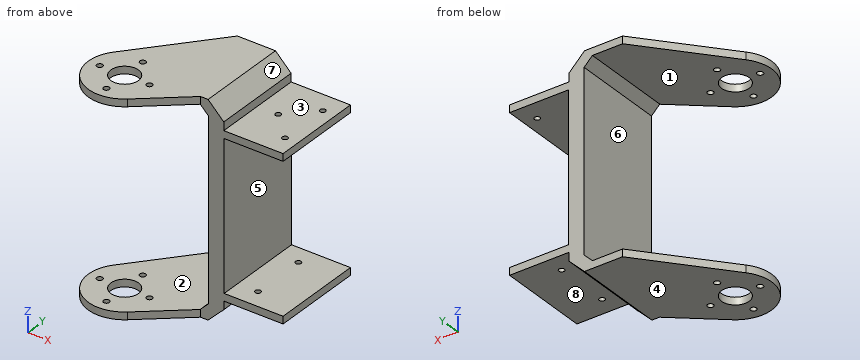
from build123d import *

# Parameters (mm, degrees)
EXTRUDE_1_DEPTH                 = 25
CUT_EXTRUDE_1_REACH             = 54.692
SKETCH_2_R                      = 0.75
CUT_EXTRUDE_1_DIRECTION_2_DEPTH = 53.691808082
EXTRUDE_2_DEPTH                 = 25
EXTRUDE_3_DEPTH                 = 2
CUT_EXTRUDE_4_DEPTH             = 73.027407742
CUT_EXTRUDE_4_DEPTH_BACK        = 73.027407742
SKETCH_6_R                      = 3.75
SKETCH_6_R_2                    = 0.8
CUT_EXTRUDE_START               = -44
SKETCH_8_R                      = 0.75
CUT_EXTRUDE_5_DEPTH             = 2


with BuildPart() as part:
    # 草图1 → 凸台-拉伸1 (new body)
    with BuildSketch(Plane(origin=(0, 0, 0), x_dir=(1, 0, 0), z_dir=(0, 1, 0))):
        Polygon((14.677419355, 32.709677419), (-1.322580645, 32.709677419), (-1.322580645, -7.290322581), (14.677419355, -7.290322581), (14.677419355, -9.290322581), (-3.322580645, -9.290322581), (-3.322580645, 34.709677419), (14.677419355, 34.709677419), align=None)
    extrude(amount=EXTRUDE_1_DEPTH)

    # 草图2 → 切除-拉伸1 (cut, up to next)
    with BuildSketch(Plane.XY.offset(9.290322581), mode=Mode.PRIVATE) as cut_extrude_1_sk1:
        with Locations(Location((4.195809336, 12.5, 0), (0, 0, 180))):
            Circle(SKETCH_2_R)
    cut_extrude_1_tool1 = extrude(cut_extrude_1_sk1.sketch, amount=-CUT_EXTRUDE_1_REACH, mode=Mode.PRIVATE) & part.part
    # 草图2 → 切除-拉伸1 (cut, up to next)
    with BuildSketch(Plane.XY.offset(9.290322581), mode=Mode.PRIVATE) as cut_extrude_1_sk2:
        with Locations(Location((11.195809336, 19.5, 0), (0, 0, 180))):
            Circle(SKETCH_2_R)
    cut_extrude_1_tool2 = extrude(cut_extrude_1_sk2.sketch, amount=-CUT_EXTRUDE_1_REACH, mode=Mode.PRIVATE) & part.part
    # 草图2 → 切除-拉伸1 (cut, up to next)
    with BuildSketch(Plane.XY.offset(9.290322581), mode=Mode.PRIVATE) as cut_extrude_1_sk3:
        with Locations(Location((11.195809336, 5.5, 0), (0, 0, 180))):
            Circle(SKETCH_2_R)
    cut_extrude_1_tool3 = extrude(cut_extrude_1_sk3.sketch, amount=-CUT_EXTRUDE_1_REACH, mode=Mode.PRIVATE) & part.part
    add(cut_extrude_1_tool1.solids().sort_by_distance((4.195809, 12.5, 9.290323))[0], mode=Mode.SUBTRACT)
    add(cut_extrude_1_tool2.solids().sort_by_distance((11.195809, 19.5, 9.290323))[0], mode=Mode.SUBTRACT)
    add(cut_extrude_1_tool3.solids().sort_by_distance((11.195809, 5.5, 9.290323))[0], mode=Mode.SUBTRACT)

    # 草图2 → 切除-拉伸1 direction 2 (cut)
    with BuildSketch(Plane.XY.offset(9.290322581)):
        with Locations(Location((4.195809336, 12.5, 0), (0, 0, 180))):
            Circle(SKETCH_2_R)
        with Locations(Location((11.195809336, 19.5, 0), (0, 0, 180))):
            Circle(SKETCH_2_R)
        with Locations(Location((11.195809336, 5.5, 0), (0, 0, 180))):
            Circle(SKETCH_2_R)
    extrude(amount=CUT_EXTRUDE_1_DIRECTION_2_DEPTH, mode=Mode.SUBTRACT)

    # 草图5 → 凸台-拉伸2 (add)
    with BuildSketch(Plane(origin=(0, 25, 0), x_dir=(1, 0, 0), z_dir=(0, 1, 0))):
        Polygon((-3.682839685, 39.209677419), (-1.432839685, 36.959677419), (-1.432839685, 34.709677419), (-3.322580645, 34.709677419), (-3.322580645, 32.459677419), (-3.322580645, 12.709677419), (-5.572580645, 12.709677419), (-5.572580645, 32.459677419), (-5.572580645, 36.959677419), (-7.822580645, 39.209677419), (-16.014767983, 39.209677419), (-16.014767983, 41.209677419), (-5.682839685, 41.209677419), align=None)
    extrude_2 = extrude(amount=-EXTRUDE_2_DEPTH)

    # 镜向1: 凸台-拉伸2 across plane
    add(extrude_2.mirror(Plane.XY.offset(-12.709677419)))

    # 草图7 → 凸台-拉伸3 (add)
    with BuildSketch(Plane(origin=(0, 0, -41.209677419), x_dir=(-1, 0, 0), z_dir=(0, 0, -1))):
        with BuildLine():
            Line((16.014767983, 25), (33.935605331, 3.642777708))
            ThreePointArc((33.935605331, 3.642777708), (33.352966922, -9.701835828), (20.008353386, -10.284474238))
            Line((20.008353386, -10.284474238), (7.751794264, 0))
            Line((7.751794264, 0), (16.014767983, 0))
            Line((16.014767983, 0), (16.014767983, 25))
        make_face()
    extrude_3 = extrude(amount=-EXTRUDE_3_DEPTH)

    # 镜向5: 凸台-拉伸3 across plane
    add(extrude_3.mirror(Plane.XY.offset(-12.709677419)))

    # 草图6 → 切除-拉伸4 (cut, two sides: drawn at the far end of the back side and taken through both)
    with BuildSketch(Plane(origin=(0, 0, -41.209677419), x_dir=(-1, 0, 0), z_dir=(0, 0, -1)).offset(-CUT_EXTRUDE_4_DEPTH_BACK)):
        with Locations((26.362741029, -2.711609936)):
            Circle(SKETCH_6_R)
        with Locations((33.112741029, -2.711609936)):
            Circle(SKETCH_6_R_2)
        with Locations((26.362741029, 4.038390064)):
            Circle(SKETCH_6_R_2)
        with Locations((19.612741029, -2.711609936)):
            Circle(SKETCH_6_R_2)
        with Locations((26.362741029, -9.461609936)):
            Circle(SKETCH_6_R_2)
    extrude(amount=CUT_EXTRUDE_4_DEPTH + CUT_EXTRUDE_4_DEPTH_BACK, mode=Mode.SUBTRACT)

    # 草图8 → 切除-拉伸5 (cut)
    with BuildSketch(Plane.XY.offset(9.290322581).offset(CUT_EXTRUDE_START)):
        with Locations((4.195809336, 20)):
            Circle(SKETCH_8_R)
        with Locations((4.195809336, 5)):
            Circle(SKETCH_8_R)
    extrude(amount=CUT_EXTRUDE_5_DEPTH, mode=Mode.SUBTRACT)


solid = part.part
Model file for the job. Use its own axes, mm. Face numbers are marked on the shaded views. A direction names the side the tool comes from. Give positions to 0.01 mm unless a question says otherwise; leave off trailing zeros. Loops run counter-clockwise (first coordinate to the right, second up) from the corner with the lowest first, then second, coordinate; pieces in that order, holes last.
1) Pull direction Z, two halves, no side cores. Call the marked faces 1, 2, 3 and 4: +Z half, -Z half, draft (parallel to the pull), parting line (faces both ways), or undercut.
2) Saw through at D-D (y = 12.5). Write the cut outline in (x, z), plus the area to 3 significant figures.
3) Saw through at B-B (z = 8.5). Write the cut outline in (x, y), plus the area to 3 significant figures.
4) Tool access for the marked faces 5, 6, 7 and 8: list every direction of +Z, -Z, +X, -X, +Y, -Y with a clear straight run to the whole face (end or side of a thin tool).
5) Saw through at C-C (x = -24). Write the cut outline in (y, z).
6) Saw through at A-A (x = 2.5). Write the cut outline in (y, z), plus the area to 3 significant figures.
7) Wall check: line 1 (X direction, y = 12.5, z = 8.2); line 2 (Z direction, x = 0, y = 20.5); line 3 (Z direction, x = -27.5, y = 6.5). Give the ranges that are in metal, low to high.
8) Flat gauge pins, fed straight in: pin 1 Ø1.2 at (x, y) = (11.2, 19.5) entering from -Z; pin 2 Ø6 at (y, z) = (4, -13) entering from -X; pin 3 Ø1.7 at (x, y) = (11.2, 5.5) entering from +Z; pin 4 Ø1.4 at (x, y) = (-26.36, 4.04) entering from -Z. Where does each tip first touch, or does it go through?
Answer block:
1. face 1: undercut
1. face 2: undercut
1. face 3: +Z half
1. face 4: -Z half
2. outline: (-26.5, -41.21) - (-5.68, -41.21) - (-1.43, -36.96) - (-1.43, -34.71) - (14.68, -34.71) - (14.68, -32.71) - (-1.32, -32.71) - (-1.32, 7.29) - (3.45, 7.29) - (3.45, 9.29) - (-1.43, 9.29) - (-1.43, 11.54) - (-5.68, 15.79) - (-26.5, 15.79) - (-26.5, 13.79) - (-7.82, 13.79) - (-5.57, 11.54) - (-5.57, -36.96) - (-7.82, -39.21) - (-26.5, -39.21) - close; (4.95, 7.29) - (14.68, 7.29) - (14.68, 9.29) - (4.95, 9.29) - close
2. area: 373 mm2
3. outline: (-5.57, 0) - (14.68, 0) - (14.68, 25) - (-5.57, 25) - close; hole circle Ø1.5 at (4.2, 12.5); hole circle Ø1.5 at (11.2, 5.5); hole circle Ø1.5 at (11.2, 19.5)
3. area: 501 mm2
4. face 5: +X, +Y, -Y
4. face 6: -X, +Y, -Y
4. face 7: +Z, +X, +Y, -Y
4. face 8: -Z, +X, +Y, -Y
5. outline: (-12.31, -41.21) - (-5.62, -41.21) - (-5.62, -39.21) - (-12.31, -39.21) - close; (-12.31, 13.79) - (-5.62, 13.79) - (-5.62, 15.79) - (-12.31, 15.79) - close; (0.2, -41.21) - (15.48, -41.21) - (15.48, -39.21) - (0.2, -39.21) - close; (0.2, 13.79) - (15.48, 13.79) - (15.48, 15.79) - (0.2, 15.79) - close
6. outline: (0, -34.71) - (25, -34.71) - (25, -32.71) - (0, -32.71) - close; (0, 7.29) - (25, 7.29) - (25, 9.29) - (0, 9.29) - close
6. area: 100 mm2
7. line 1: x = -5.57 to 3.45, 4.95 to 14.68
7. line 2: z = -34.71 to -32.71, 7.29 to 9.29
7. line 3: z = -41.21 to -39.21, 13.79 to 15.79
8. pin 1: stops at z = -34.71
8. pin 2: stops at x = -5.57
8. pin 3: stops at z = 9.29
8. pin 4: passes through
